```python
from build123d import *

# Parameters (mm, degrees)
F1_DEPTH  = 25
F3_DEPTH  = 70
F5_DEPTH  = 10
F6_R      = 15
F7_DEPTH  = 10
F8_R      = 7.44
F9_DEPTH  = 25.001
F11_DEPTH = 20
F13_R     = 35.5
F14_DEPTH = 130
F15_R     = 20.5
F16_DEPTH = 223.001
F18_R     = 35.5
F19_DEPTH = 130
F20_R     = 21.5
F21_DEPTH = 210.001
F22_SIZE2 = 2
F22_SIZE  = 2


with BuildPart() as f1:
    # F0 (on Top) → F1 (new body)
    with BuildSketch(Plane.XY):
        with BuildLine():
            Line((-190, 0), (-10, 0))
            ThreePointArc((-10, 0), (-2.9289321881, 2.9289321881), (0, 10))
            Line((0, 10), (0, 203))
            ThreePointArc((0, 203), (-2.9289321881, 210.0710678119), (-10, 213))
            Line((-10, 213), (-190, 213))
            ThreePointArc((-190, 213), (-197.0710678119, 210.0710678119), (-200, 203))
            Line((-200, 203), (-200, 10))
            ThreePointArc((-200, 10), (-197.0710678119, 2.9289321881), (-190, 0))
        make_face()
    extrude(amount=F1_DEPTH)

    # F2 (on face) → F3 (join)
    with BuildSketch(Plane.XY.offset(25)):
        with BuildLine():
            Line((0, 155), (0, 170))
            Line((0, 170), (-80, 170))
            ThreePointArc((-80, 170), (-106.3603896932, 106.3603896932), (-170, 80))
            Line((-170, 80), (-170, 0))
            Line((-170, 0), (-155, 0))
            Line((-155, 0), (-155, 66.0769515459))
            ThreePointArc((-155, 66.0769515459), (-95.7537879754, 95.7537879754), (-66.0769515459, 155))
            Line((-66.0769515459, 155), (0, 155))
        make_face()
    extrude(amount=F3_DEPTH)

    # F4 (on face) → F5 (join)
    with BuildSketch(Plane.XY.offset(25)):
        with BuildLine():
            Line((0, 60), (-45, 60))
            ThreePointArc((-45, 60), (-55.6066017178, 55.6066017178), (-60, 45))
            Line((-60, 45), (-60, 0))
            Line((-60, 0), (-10, 0))
            ThreePointArc((-10, 0), (-2.9289321881, 2.9289321881), (0, 10))
            Line((0, 10), (0, 60))
        make_face()
    extrude(amount=F5_DEPTH)

    # F6 (on face) → F7 (cut)
    with BuildSketch(Plane.XY.offset(35)):
        with Locations((-30, 30)):
            Circle(F6_R)
    extrude(amount=-F7_DEPTH, mode=Mode.SUBTRACT)

    # F8 (on face) → F9 (cut, through all)
    with BuildSketch(Plane.XY.offset(25)):
        with Locations((-30, 30)):
            Circle(F8_R)
    extrude(amount=-F9_DEPTH, mode=Mode.SUBTRACT)

    # F10 (on face) → F11 (cut)
    with BuildSketch(Plane.XY.offset(25)):
        with BuildLine():
            ThreePointArc((-19, 69), (-11.9289321881, 71.9289321881), (-9, 79))
            Line((-9, 79), (-9, 136))
            ThreePointArc((-9, 136), (-11.9289321881, 143.0710678119), (-19, 146))
            Line((-19, 146), (-50.7523585139, 146))
            ThreePointArc((-50.7523585139, 146), (-56.7765034807, 143.981834214), (-60.369103795, 138.7419354839))
            ThreePointArc((-60.369103795, 138.7419354839), (-89.3898269447, 89.3898269447), (-138.7419354839, 60.369103795))
            ThreePointArc((-138.7419354839, 60.369103795), (-143.981834214, 56.7765034807), (-146, 50.7523585139))
            Line((-146, 50.7523585139), (-146, 19))
            ThreePointArc((-146, 19), (-143.0710678119, 11.9289321881), (-136, 9))
            Line((-136, 9), (-79, 9))
            ThreePointArc((-79, 9), (-71.9289321881, 11.9289321881), (-69, 19))
            Line((-69, 19), (-69, 45))
            ThreePointArc((-69, 45), (-61.9705627485, 61.9705627485), (-45, 69))
            Line((-45, 69), (-19, 69))
        make_face()
    extrude(amount=-F11_DEPTH, mode=Mode.SUBTRACT)

    # F13 (on offset) → F14 (join)
    with BuildSketch(Plane.XZ.offset(10)):
        with Locations((-162.5, 95)):
            Circle(F13_R)
    extrude(amount=-F14_DEPTH)

    # F15 (on face) → F16 (cut, through all)
    with BuildSketch(Plane.XZ.offset(10)):
        with Locations((-162.5, 95)):
            Circle(F15_R)
    extrude(amount=-F16_DEPTH, mode=Mode.SUBTRACT)

    # F18 (on offset) → F19 (join)
    with BuildSketch(Plane.YZ.offset(10)):
        with Locations((162.5, 95)):
            Circle(F18_R)
    extrude(amount=-F19_DEPTH)

    # F20 (on face) → F21 (cut, through all)
    with BuildSketch(Plane.YZ.offset(10)):
        with Locations((162.5, 95)):
            Circle(F20_R)
    extrude(amount=-F21_DEPTH, mode=Mode.SUBTRACT)

    # F22
    f22_edges = [f1.edges().sort_by_distance(p)[0] for p in [
        (-183, -10, 95),
        (-183, 120, 95),
        (10, 141, 95),
        (-120, 141, 95),
    ]]
    chamfer(f22_edges, length=F22_SIZE, length2=F22_SIZE2)


solid = f1.part
```
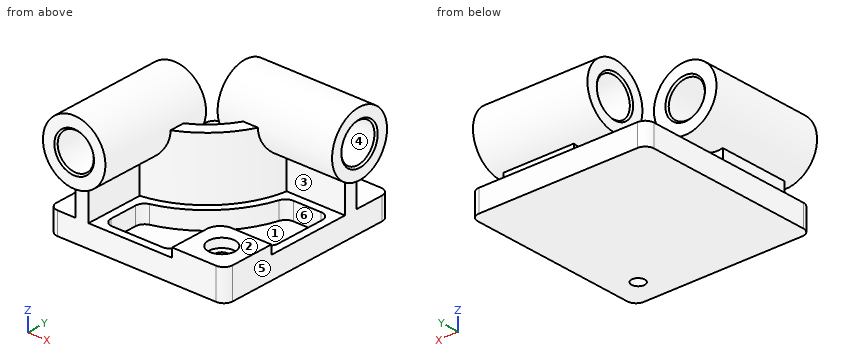
The listing builds one solid part. Answer for the finished solid, in the listing's coordinates (mm). Face numbers are marked on the shaded views. A direction names the side the tool comes from. Round coordinates to 2 decimals unless told otherwise and drop trailing zeros. Order: outer loops, then holes, each group sorted by start corner. A loop starts at its lowest first (then second) coordinate and runs counter-clockwise, first axis right, second up. Notation, with made-up numbers: (72.25, 34.5) - (90.25, 34.5) arc R21 ccw to (90.25, 72.5) - close; hole circle Ø4 at (85.25, -29.75). An arc over 180 degrees is marked (long way). Put each result on its own line as item: value. Start each with the question number.
(1) Straight lines are drawn through the part: probe 1 along Y at (x, z) = (-30, 18); probe 2 along Z at (x, y) = (-105.5, 160.5); probe 3 along X at (y, z) = (34, 10). For each, find the intervals that lie inside material, in ascending order. Write a range as from..to.
(2) Find section A-A (y = 30). Give the vertices of the cut face in (x, z).
(3) Find section C-C (y = 107.5). Give the vertices of the cut face in (x, z).
(4) Find section D-D (x = -84). Give the vertices of the cut face in (y, z), plus the area to 3 significant figures.
(5) Determine the mould class of the marked faces 4, 5 and 6 for opening direction X: released by +X, released by -X, zero draft, split by the parting line, or undercut.
(6) Given P1, Ø10, axis at x = -111.5, y = 50.5, coming from the +Z side; P2, Ø4, axis at x = -41, z = 72, coming from the +Y side; P3, Ø17.5, axis at x = -57, z = 40, coming from the +Y side, each flat-ended and moving along its own axis, determine where each tip first touches the part or whether it passes through.
(7) Find section B-B (x = -30). Give the vertices of the cut face in (y, z).
(8) For the marked faces 1, 2 and 3, determine the directions among +Z, -Z, +X, -X, +Y, -Y from which every point of the face is accessible in a straight line to the end or side of a thin tool.
Reply:
1. probe 1: 0..22.56, 37.44..69, 146..213
1. probe 2: 0..25, 59.56..73.59, 116.41..130.44
1. probe 3: -200..-146, -69..-36.27, -23.73..0
2. outline: (-200, 0) - (-37.44, 0) - (-37.44, 25) - (-45, 25) - (-45, 35) - (-60, 35) - (-60, 25) - (-69, 25) - (-69, 5) - (-146, 5) - (-146, 25) - (-155, 25) - (-155, 60.3) arc R35.5 ccw (long way) to (-170, 60.3) - (-170, 25) - (-200, 25) - close; (-22.56, 0) - (0, 0) - (0, 35) - (-15, 35) - (-15, 25) - (-22.56, 25) - close; hole circle Ø41 at (-162.5, 95)
3. outline: (-200, 0) - (0, 0) - (0, 25) - (-9, 25) - (-9, 5) - (-74.66, 5) - (-74.66, 25) - (-85.63, 25) - (-85.63, 95) - (-105.24, 95) - (-105.24, 25) - (-200, 25) - close; circle Ø71 at (-162.5, 95); hole circle Ø41 at (-162.5, 95)
4. outline: (0, 0) - (213, 0) - (213, 25) - (143.47, 25) - (143.47, 65.03) arc R35.5 ccw (long way) to (127, 95) - (109.76, 95) - (109.76, 25) - (95.17, 25) - (95.17, 5) - (9, 5) - (9, 25) - (0, 25) - close; hole circle Ø43 at (162.5, 95)
4. area: 8,120 mm^2
5. face 4: zero draft
5. face 5: released by +X
5. face 6: undercut
6. P1: z = 5
6. P2: y = 191.12
6. P3: y = 170
7. outline: (0, 0) - (22.56, 0) - (22.56, 25) - (15, 25) - (15, 35) - (0, 35) - close; (37.44, 0) - (213, 0) - (213, 25) - (170, 25) - (170, 60.3) arc R35.5 ccw (long way) to (155, 60.3) - (155, 25) - (146, 25) - (146, 5) - (69, 5) - (69, 25) - (60, 25) - (60, 35) - (45, 35) - (45, 25) - (37.44, 25) - close; hole circle Ø43 at (162.5, 95)
8. face 1: none
8. face 2: +Z, +X, -Y
8. face 3: +X
